Design review of the part shown in the three views and the two pictorial views. Dimensions are in mm from the part's minimum x, y and z. Coordinates: 2 decimals unless noted, no trailing zeros. Order: outer loops, then holes, each group sorted by start corner. A loop starts at its lowest first (then second) coordinate and runs counter-clockwise, first axis right, second up. Notation, with made-up numbers: M 63.25,60 L 87.25,60 A15 cw 87.25,82 Z; hole C 44.25,21.5 d5. An arc over 180 degrees is marked long. Use CSV: the item, a comma, the result in double quotes.
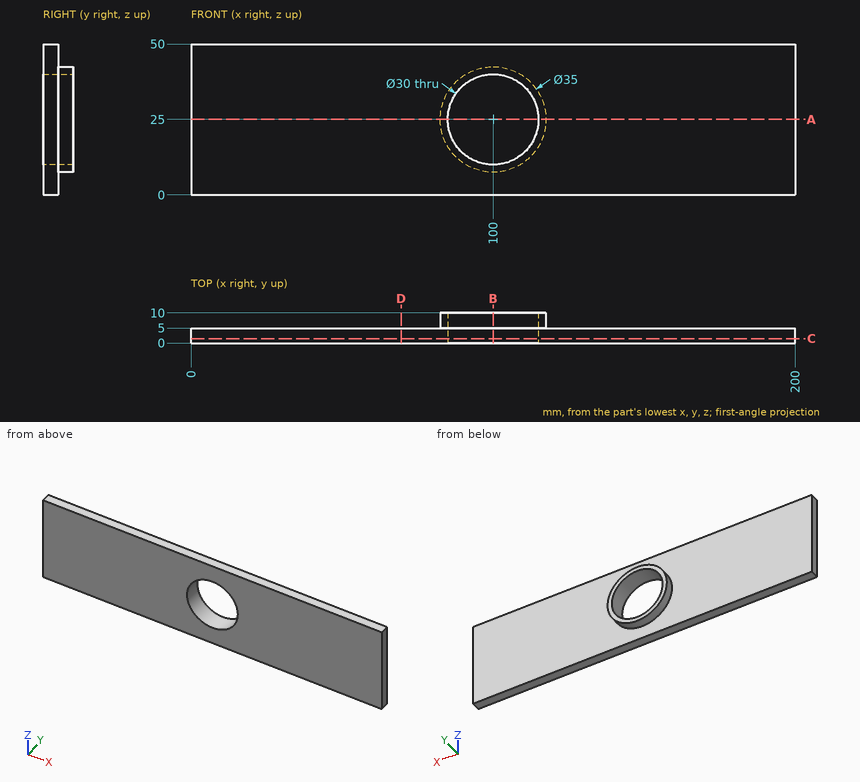
(1) Add section A-A on z = 25. State the section outline as (x, y) points, and give its area (3 significant figures).
The answers:
outline,"M 0,0 L 85,0 L 85,10 L 82.5,10 L 82.5,5 L 0,5 Z; M 115,0 L 200,0 L 200,5 L 117.5,5 L 117.5,10 L 115,10 Z"
area,"875 mm2"
(2) Wall thickness on probe 1 along X at (y, z) = (6.75, 25); probe 2 along X at (y, z) = (2.25, 25); probe 3 along Y at (x, z) = (171.5, 29): over which ranges is each line inside the solid? List them lowest first.
The answers:
probe 1,"x = 82.5 to 85, 115 to 117.5"
probe 2,"x = 0 to 85, 115 to 200"
probe 3,"y = 0 to 5"
(3) Add section B-B on x = 100. State the section outline as (y, z) points.
The answers:
outline,"M 0,0 L 5,0 L 5,7.5 L 10,7.5 L 10,10 L 0,10 Z; M 0,40 L 10,40 L 10,42.5 L 5,42.5 L 5,50 L 0,50 Z"
(4) Add section D-D on x = 69.5. State the section outline as (y, z) points, and give its area (3 significant figures).
The answers:
outline,"M 0,0 L 5,0 L 5,50 L 0,50 Z"
area,"250 mm2"
(5) Add section C-C on y = 1.5. State the section outline as (x, z) points.
The answers:
outline,"M 0,0 L 200,0 L 200,50 L 0,50 Z; hole C 100,25 d30"
(6) Clearance check with a flat-ended pin moving along its axis: P1, Ø8, axis at x = 23.5, z = 28, coming from the +Y side. State where the tip first meets the part, or that it passes through.
The answers:
P1,"stops at y = 5"
